Read the model definition and answer for the solid it produces. Units are mm, in the model's axes. Face numbers are marked on the shaded views. A direction names the side the tool comes from. Coordinates: 2 decimals unless noted, no trailing zeros. Loops run counter-clockwise (first coordinate to the right, second up) from the corner with the lowest first, then second, coordinate; pieces in that order, holes last. Notation, with made-up numbers: M 27.25,68.25 L 36.25,68.25 A13 ccw 36.25,78.25 Z; hole C -35,18.25 d4. An arc over 180 degrees is marked long. One line per item, written item: value. Start each with the question number.
1. The part is cut by section A-A (z = 6). Write down the section's boundary in (x, y), then the cut area to 3 significant figures.
2. The part is cut by section B-B (x = -1.5). Write down the section's boundary in (y, z).
3. The part is cut by section D-D (x = -17.5). Write down the section's boundary in (y, z), then the cut area to 3 significant figures.
4. Determine the mould class of the marked faces 1, 2 and 3 for opening direction X: +X half, -X half, draft (parallel to the pull), parting line (faces both ways), or undercut.
5. For the marked faces 4, 5 and 6, determine the directions among +Z, -Z, +X, -X, +Y, -Y from which every point of the face is accessible in a straight line to the end or side of a thin tool.
6. Consider probe 1 along Z at (x, y) = (-19.5, 5.9); probe 2 along X at (y, z) = (6.2, -3.2); probe 3 along Z at (x, y) = (1.5, 0). Determine where each line is inside the solid, lowest interval first.
7. The part is cut by section C-C (y = -5). Write down the section's boundary in (x, z).
8. Flat-ended cylindrical pins translate along their axes: pin 1 (1.8 mm diameter, centred on x = -19.5, z = 16, fed in from -Y); pin 2 (8 mm diameter, centred on x = -2, y = -2.5, fed in from +Z); pin 3 (1 mm diameter, centred on y = 6.5, z = 10, fed in from -X); pin 4 (8 mm diameter, centred on x = 0, y = -1.5, fed in from -Z). Find the tip coordinate at first contact, or state that the pin passes through.
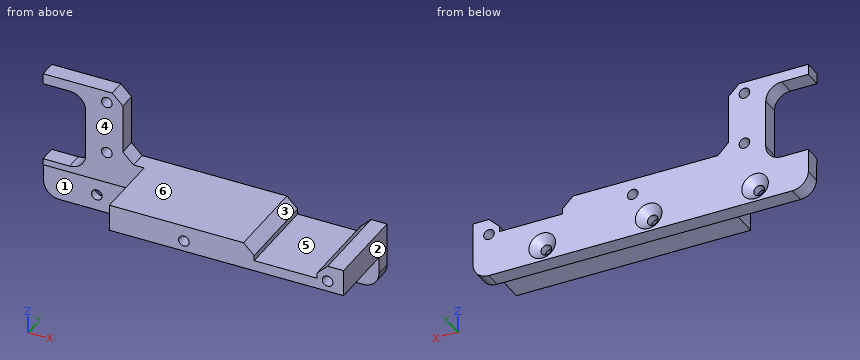
Autodesk Inventor part; units mm, degrees
ref_plane "YZ Plane" through (0, 0, 0) normal (1, 0, 0) x (0, 1, 0)
ref_plane "XZ Plane" through (0, 0, 0) normal (0, 1, 0) x (-1, 0, 0)
ref_plane "XY Plane" through (0, 0, 0) normal (0, 0, 1) x (1, 0, 0)
sketch "Sketch1" plane through (0, 0, 0) normal (0, 0, 1) x (1, 0, 0)
  line L0 (-31.5, 8) -> (31.5, 8)
  line L1 (31.5, 8) -> (31.5, -8)
  line L2 (31.5, -8) -> (-31.5, -8)
  line L3 (-31.5, -8) -> (-31.5, 8)
  point P0 (0, 0)
  dimension "d0" = 16
  dimension "d1" = 8
  dimension "d2" = 63
  dimension "d3" = 31.5
extrude "Extrusion1" add sketch "Sketch1" along normal blind 5
sketch "Sketch2" plane through (-31.5, 8, 0) normal (0, 1, 0) x (1, 0, 0)
  line L0 (0, 0) -> (0, -5)
  line L1 (63, 0) -> (0, 0)
  circle A0 centre (33, -2) radius 1
  circle A1 centre (60, -2) radius 1
  point P0 (31.5, 0)
  dimension "d6" = 33
  dimension "d7" = 60
  dimension "d8" = 2
  dimension "d9" = 2
  dimension "d10" = 2
  dimension "d11" = 2
extrude "Extrusion2" cut sketch "Sketch2" against normal blind 16
sketch "Sketch4" plane through (0, 0, 5) normal (0, 0, 1) x (1, 0, 0)
  line L0 (-31.5, -8) -> (31.5, -8)
  line L1 (-31.5, -8) -> (-12.5, -8)
  line L2 (-12.5, -8) -> (-12.5, 4.8)
  line L3 (-12.5, 4.8) -> (-31.5, 4.8)
  line L4 (-31.5, 4.8) -> (-31.5, -8)
  line L5 (31.5, 8) -> (-31.5, 8)
  point P0 (0, 0)
  dimension "d24" = 19
  dimension "d25" = 3.2
extrude "Extrusion4" cut sketch "Sketch4" against normal blind 5
sketch "Sketch5" plane through (-31.5, 8, 0) normal (0, 1, 0) x (1, 0, 0)
  line L0 (0, 0) -> (0, -5)
  line L1 (0, -1.2) -> (8, -1.2)
  line L2 (8, -1.2) -> (8, -5)
  line L3 (8, -5) -> (0, -5)
  line L4 (0, -5) -> (0, -1.2)
  line L5 (63, 0) -> (0, 0)
  line L6 (63, -5) -> (0, -5)
  point P0 (31.5, 0)
  dimension "d28" = 1.2
  dimension "d29" = 8
extrude "Extrusion5" cut sketch "Sketch5" against normal blind 5
sketch "Sketch6" plane through (-31.5, 8, 0) normal (0, 1, 0) x (1, 0, 0)
  line L0 (8, -1.2) -> (0, -1.2)
  line L1 (0, -1.2) -> (10, -1.2)
  line L2 (10, -1.2) -> (10, -18.2)
  line L3 (10, -18.2) -> (0, -18.2)
  line L4 (0, -18.2) -> (0, -1.2)
  line L5 (8, -5) -> (10, -5)
  line L6 (10, -5) -> (10, -18.2)
  line L7 (10, -18.2) -> (8, -18.2)
  line L8 (8, -18.2) -> (8, -5)
  line L9 (0, -18.2) -> (8, -18.2)
  line L10 (8, -18.2) -> (8, -16.2)
  line L11 (8, -16.2) -> (0, -16.2)
  line L12 (0, -16.2) -> (0, -18.2)
  line L13 (63, -5) -> (8, -5)
  line L14 (8, -1.2) -> (8, -5)
  point P0 (31.5, 0)
  point P1 (10, -5)
  point P2 (0, -16.2)
  dimension "d32" = 2
  dimension "d33" = 15
  dimension "d34" = 2
extrude "Extrusion6" add sketch "Sketch6" against normal blind 3.2 contours L5 L2 L3 L8 | L11 L8 L3 L4
sketch "Sketch7" plane through (-31.5, 8, 0) normal (0, 1, 0) x (1, 0, 0)
  line L0 (0, 0) -> (0, -1.2)
  line L1 (0, -16.2) -> (0, -18.2)
  line L2 (63, 0) -> (0, 0)
  circle A0 centre (12, -6) radius 1
  circle A1 centre (12, -16) radius 1
  line L3 (10, -18.2) -> (0, -18.2)
  line L4 (10, -5) -> (19, -5)
  line L5 (10, -18.2) -> (15, -18.2)
  line L6 (15, -18.2) -> (15, -5)
  line L7 (15, -5) -> (10, -5)
  line L8 (10, -5) -> (10, -18.2)
  point P0 (31.5, 0)
  point P1 (12, -5)
  dimension "d37" = 12
  dimension "d38" = 12
  dimension "d39" = 16
  dimension "d40" = 6
  dimension "d41" = 2
  dimension "d42" = 2
  dimension "d43" = 5
extrude "Extrusion7" add sketch "Sketch7" against normal blind 3.2
chamfer "Chamfer1" distance 2 angle 45 2 edges at (-16.5, 6.4, 18.2) (-16.5, 6.4, 5)
fillet "Fillet1" radius 3 2 edges at (-23.5, 6.4, 1.2) (-23.5, 6.4, 16.2)
sketch "Sketch10" plane through (-31.5, 8, 0) normal (0, 1, 0) x (1, 0, 0)
  line L0 (63, -5) -> (17, -5)
  line L1 (46.2, -5) -> (58, -5)
  line L2 (58, -5) -> (58, -2)
  line L3 (58, -2) -> (46.2, -2)
  line L4 (46.2, -2) -> (46.2, -5)
  line L5 (0, 0) -> (0, -1.2)
  line L6 (63, 0) -> (0, 0)
  point P0 (31.5, 0)
  dimension "d73" = 46.2
  dimension "d74" = 58
  dimension "d75" = 2
extrude "Extrusion9" cut sketch "Sketch10" against normal blind 16
chamfer "Chamfer2" distance 2 angle 45 2 edges at (14.7, 0, 5) (26.5, 0, 5)
sketch "Sketch11" plane through (-31.5, 8, 0) normal (0, 1, 0) x (1, 0, 0)
  line L0 (63, 0) -> (0, 0)
  line L1 (0, 0) -> (63, 0)
  line L2 (63, 0) -> (63, 6.2)
  line L3 (63, 6.2) -> (0, 6.2)
  line L4 (0, 6.2) -> (0, 0)
  line L5 (63, 0) -> (63, -5)
  point P0 (31.5, 0)
  dimension "d81" = 6.2
extrude "Extrusion10" add sketch "Sketch11" against normal blind 3
sketch "Sketch12" plane through (-31.5, 8, 18.2) normal (0, 1, 0) x (1, 0, 0)
  line L0 (63, 24.4) -> (0, 24.4)
  line L1 (0, 24.4) -> (0, 17)
  point P0 (31.5, 18.2)
  point P1 (10, 21.4)
  point P2 (30, 21.4)
  point P3 (50, 21.4)
  dimension "d84" = 3
  dimension "d85" = 3
  dimension "d86" = 3
  dimension "d87" = 20
  dimension "d88" = 20
  dimension "d89" = 10
hole "Hole2" at (-21.5, 8, -3.2) at (-1.5, 8, -3.2) at (18.5, 8, -3.2) direction (0, -1, 0) diameter 2 depth 5 tip angle 118 countersink diameter 5 countersink angle 90
fillet "Fillet2" radius 3 2 edges at (31.5, 6.5, -6.2) (-31.5, 6.5, -6.2)
properties part number "bridge_structure_A"
Answer block:
1. outline: M -23.5,4.8 L -20.5,4.8 L -20.5,8 L -23.5,8 Z; M -18.5,4.8 L -15.5,4.8 L -15.5,8 L -18.5,8 Z
1. area: 19.2 mm2
2. outline: M -8,0 L 5,0 L 5,-2.2 L 6.5,-2.2 L 8,-0.7 L 8,5 L -8,5 Z; M 5,-6.2 L 8,-6.2 L 8,-5.7 L 6.5,-4.2 L 5,-4.2 Z
3. outline: M 4.8,0 L 5,0 L 5,-6.2 L 8,-6.2 L 8,17.2 L 4.8,17.2 Z
3. area: 73.6 mm2
4. face 1: draft
4. face 2: +X half
4. face 3: undercut
5. face 4: +Z, -Z, -X, -Y
5. face 5: +Z, +Y, -Y
5. face 6: +Z, +X, +Y, -Y
6. probe 1: z = -6.2 to 5, 7 to 15, 17 to 18.2
6. probe 2: x = -31.5 to -22.5, -20.5 to -2.5, -0.5 to 17.5, 19.5 to 31.5
6. probe 3: z = 0 to 1, 3 to 5
7. outline: M -12.5,0 L 31.5,0 L 31.5,5 L 28.5,5 L 26.5,3 L 26.5,2 L 14.7,2 L 14.7,3 L 12.7,5 L -12.5,5 Z; hole C 1.5,2 d2; hole C 28.5,2 d2
8. pin 1: passes through
8. pin 2: stops at z = 5
8. pin 3: stops at x = -23.5
8. pin 4: stops at z = 0
